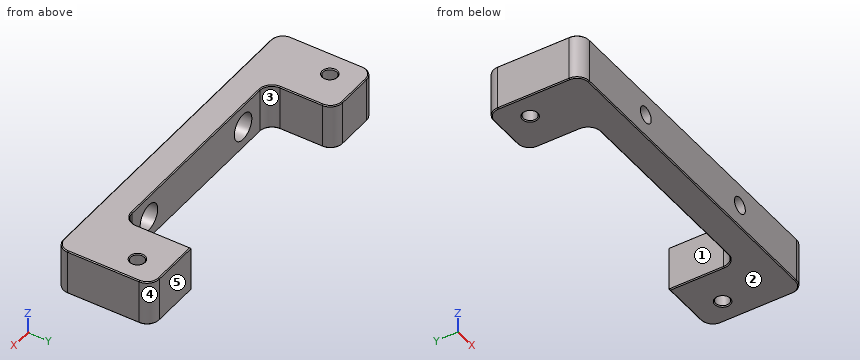
from build123d import *

# Parameters (mm, degrees)
SKETCH1_W                       = 71.12
SKETCH1_H                       = 20
EXTRUDE1_DEPTH                  = 9.525
SKETCH2_W                       = 45.72
SKETCH2_H                       = 13.97
EXTRUDE2_DEPTH                  = 10.525
HOLE1_D                         = 3.4544
HOLE1_CBORE_D                   = 5.588
HOLE1_CBORE_DEPTH               = 3.048
F_4_40_TAPPED_HOLE1_D           = 2.2606
F_4_40_TAPPED_HOLE1_DEPTH       = 12.6746
F_4_40_TAPPED_HOLE1_CBORE_D     = 2.8448
F_4_40_TAPPED_HOLE1_CBORE_DEPTH = 10.7696
F_4_40_TAPPED_HOLE1_TIP         = 0.679152758
FILLET1_R                       = 2.54
CHAMFER1_SIZE                   = 0.2


with BuildPart() as part:
    # Sketch1 → Extrude1 (new body)
    with BuildSketch(Plane.XY):
        with Locations((-35.56, 10)):
            Rectangle(SKETCH1_W, SKETCH1_H)
    extrude(amount=EXTRUDE1_DEPTH)

    # Sketch2 → Extrude2 (cut, through all)
    with BuildSketch(Plane.XY.offset(9.525)):
        with Locations((-35.56, 13.015)):
            Rectangle(SKETCH2_W, SKETCH2_H)
    extrude(amount=-EXTRUDE2_DEPTH, mode=Mode.SUBTRACT)

    # Hole1 (through all)
    with Locations(Plane(origin=(-50.56, 6.03, 4.7625), x_dir=(0, 0, 1), z_dir=(0, 1, 0))):
        with Locations((0, 0), (0, 30)):
            CounterBoreHole(HOLE1_D / 2, HOLE1_CBORE_D / 2, HOLE1_CBORE_DEPTH)

    # #4-40 Tapped Hole1
    with Locations(Plane(origin=(-66.2305, 13.9, 9.525), x_dir=(1, 0, 0), z_dir=(0, 0, 1))):
        with Locations((0, 0), (61.341, 0)):
            CounterBoreHole(F_4_40_TAPPED_HOLE1_D / 2, F_4_40_TAPPED_HOLE1_CBORE_D / 2, F_4_40_TAPPED_HOLE1_CBORE_DEPTH, depth=F_4_40_TAPPED_HOLE1_DEPTH)
            with Locations((0, 0, -(F_4_40_TAPPED_HOLE1_DEPTH + F_4_40_TAPPED_HOLE1_TIP / 2))):  # 118° drill point
                Cone(0, F_4_40_TAPPED_HOLE1_D / 2, F_4_40_TAPPED_HOLE1_TIP, mode=Mode.SUBTRACT)

    # Fillet1
    fillet1_edges = [part.edges().sort_by_distance(p)[0] for p in [
        (-58.42, 6.03, 4.7625),
        (-58.42, 20, 4.7625),
        (-12.7, 6.03, 4.7625),
        (0, 0, 4.7625),
        (-71.12, 0, 4.7625),
        (-71.12, 20, 4.7625),
        (0, 20, 4.7625),
    ]]
    fillet(fillet1_edges, radius=FILLET1_R)

    # Chamfer1
    chamfer1_edges = [part.edges().sort_by_distance(p)[0] for p in [
        (-6.3119, 13.9, 0),
        (-6.3119, 13.9, 9.525),
        (-67.6529, 13.9, 0),
        (-67.6529, 13.9, 9.525),
        (-35.56, 0, 0),
        (-35.56, 0, 9.525),
        (-64.77, 20, 0),
        (-58.42, 13.015, 0),
        (-35.56, 6.03, 0),
        (-12.7, 14.285, 0),
        (-7.62, 20, 0),
        (0, 10, 0),
        (-71.12, 10, 0),
        (-0.743948776, 19.256051224, 0),
        (-59.163948776, 19.256051224, 0),
        (-70.376051224, 19.256051224, 0),
        (-0.743948776, 0.743948776, 0),
        (-70.376051224, 0.743948776, 0),
        (-71.12, 10, 9.525),
        (-58.42, 13.015, 9.525),
        (-64.77, 20, 9.525),
        (0, 10, 9.525),
        (-7.62, 20, 9.525),
        (-12.7, 14.285, 9.525),
        (-35.56, 6.03, 9.525),
        (-0.743948776, 19.256051224, 9.525),
        (-59.163948776, 19.256051224, 9.525),
        (-70.376051224, 19.256051224, 9.525),
        (-0.743948776, 0.743948776, 9.525),
        (-70.376051224, 0.743948776, 9.525),
        (-13.443948776, 6.773948776, 9.525),
        (-13.443948776, 6.773948776, 0),
        (-57.676051224, 6.773948776, 9.525),
        (-57.676051224, 6.773948776, 0),
    ]]
    chamfer(chamfer1_edges, length=CHAMFER1_SIZE)


solid = part.part
Geometry: final body of the model. Coordinates: model frame, mm. Face numbers are marked on the shaded views. A direction names the side the tool comes from. Round coordinates to 2 decimals unless told otherwise and drop trailing zeros. Put each result on its own line as item: value. Start each with the question number.
(1) Section query A-A (y = 13.9). State how many separate pieces and enclosed holes the cut face has, then the cut area to 3 significant figures.
(2) Material intervals for line 1 along X through (y, z) = (9.75, 1.5); line 2 along X through (y, z) = (12.75, 6); line 3 along X through (y, z) = (5.5, 3.5), sorted ascending. Write a range as [from, to].
(3) Contact query for flat-ended pins moving along their axis: pin 1 Ø4.5 at (x, z) = (-41.5, 5) entering from +Y; pin 2 Ø4.5 at (x, z) = (-50.56, 4.76) entering from -Y; pin 3 Ø5 at (x, z) = (-50.56, 4.76) entering from +Y. Output: stop coordinate, or through.
(4) Draft query along X for the marked faces 3, 4 and 5. Return one class per face: +X half, -X half, draft (parallel to the pull), parting line (faces both ways), or undercut.
(5) Set-up query: the marked faces 1 and 2. Return all of +Z, -Z, +X, -X, +Y, -Y with unobstructed straight access to the full face (end or side cutting, diameter ignored); none if empty.
Findings below:
1. separate pieces: 4
1. enclosed holes: 0
1. area: 187 mm2
2. line 1: x = [-71.12, -58.42], [-12.7, 0]
2. line 2: x = [-71.12, -67.07], [-65.39, -58.42], [-12.7, -5.73], [-4.05, 0]
2. line 3: x = [-71.12, -53.05], [-48.07, -23.05], [-18.07, 0]
3. pin 1: stops at y = 6.03
3. pin 2: stops at y = 0
3. pin 3: stops at y = 2.98
4. face 3: undercut
4. face 4: +X half
4. face 5: draft
5. face 1: +Z, -Z, +Y
5. face 2: -Z, +X, -X, +Y, -Y
